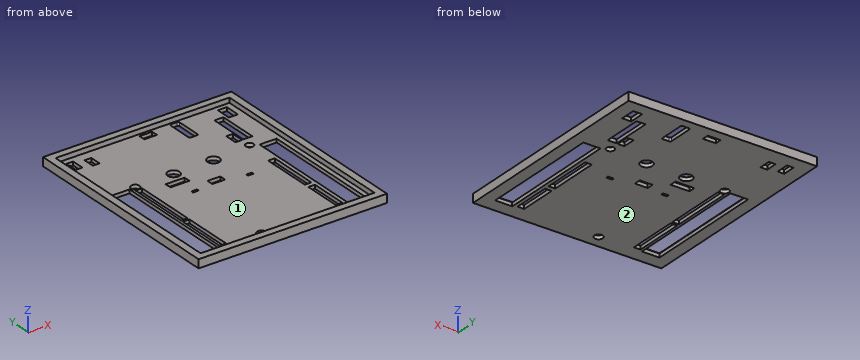
from build123d import *

# Parameters (mm, degrees)
SKETCH1_W           = 78
SKETCH1_H           = 88.5
SKETCH1_W_2         = 72
SKETCH1_H_2         = 82.5
BOSS_EXTRUDE1_DEPTH = 2
SKETCH2_W           = 78
SKETCH2_H           = 88.5
BOSS_EXTRUDE2_DEPTH = 1.5
SKETCH7_W           = 7.279998142
SKETCH7_H           = 50.36
SKETCH7_W_2         = 7.079999996
SKETCH7_H_2         = 50.160000192
CUT_EXTRUDE1_DEPTH  = 15
SKETCH8_R           = 1.738
SKETCH8_R_2         = 1.6
CUT_EXTRUDE2_DEPTH  = 10
SKETCH9_R           = 2.464925529
CUT_EXTRUDE3_DEPTH  = 10
SKETCH11_W          = 5.279999902
SKETCH11_H          = 2.74
SKETCH11_W_2        = 2.74
SKETCH11_H_2        = 5.28
SKETCH11_W_3        = 7.819999902
SKETCH11_W_4        = 5.280000098
SKETCH11_H_3        = 2.739999805
CUT_EXTRUDE4_DEPTH  = 10
SKETCH10_W          = 2.740000978
SKETCH10_H          = 25.907999907
SKETCH10_W_2        = 2.739999218
SKETCH10_H_2        = 20.828000093
SKETCH10_W_3        = 2.73999941
SKETCH10_H_3        = 15.594000099
SKETCH10_W_4        = 3.739999409
SKETCH10_H_4        = 16.440000004
SKETCH10_W_5        = 2.739999409
SKETCH10_H_5        = 15.440000004
SKETCH10_W_6        = 3.739999801
SKETCH10_H_6        = 6.280000102
SKETCH10_W_7        = 2.739999801
SKETCH10_H_7        = 5.280000102
CUT_EXTRUDE5_DEPTH  = 10
CUT_EXTRUDE6_DEPTH  = 10


with BuildPart() as part:
    # Sketch1 → Boss-Extrude1 (new body)
    with BuildSketch(Plane.XY):
        with Locations((19.784172662, -18.690647482)):
            Rectangle(SKETCH1_W, SKETCH1_H)
        with Locations((19.784172662, -18.690647482)):
            Rectangle(SKETCH1_W_2, SKETCH1_H_2, mode=Mode.SUBTRACT)
    extrude(amount=BOSS_EXTRUDE1_DEPTH)

    # Sketch2 → Boss-Extrude2 (add)
    with BuildSketch(Plane(origin=(0, 0, 0), x_dir=(-1, 0, 0), z_dir=(0, 0, -1))):
        with Locations((-19.784172662, -18.690647482)):
            Rectangle(SKETCH2_W, SKETCH2_H)
    extrude(amount=BOSS_EXTRUDE2_DEPTH)

    # Sketch7 → Cut-Extrude1 (cut)
    with BuildSketch(Plane.XY):
        with Locations((-10.583804942, -31.990645157)):
            Rectangle(SKETCH7_W, SKETCH7_H)
        with Locations((50.276195985, -32.090647407)):
            Rectangle(SKETCH7_W_2, SKETCH7_H_2)
    extrude(amount=-CUT_EXTRUDE1_DEPTH, mode=Mode.SUBTRACT)

    # Sketch8 → Cut-Extrude2 (cut)
    with BuildSketch(Plane(origin=(0, 0, -1.5), x_dir=(-1, 0, 0), z_dir=(0, 0, -1))):
        with Locations((-10.782151243, -57.440646574)):
            Circle(SKETCH8_R)
        with Locations((4.457850712, -6.640647161)):
            Circle(SKETCH8_R)
        with Locations((-43.802149239, -5.370645303)):
            Circle(SKETCH8_R_2)
    extrude(amount=-CUT_EXTRUDE2_DEPTH, mode=Mode.SUBTRACT)

    # Sketch9 → Cut-Extrude3 (cut)
    with BuildSketch(Plane(origin=(0, 0, -1.5), x_dir=(-1, 0, 0), z_dir=(0, 0, -1))):
        with Locations((-27.927151828, -6.640645914)):
            Circle(SKETCH9_R)
        with Locations((-11.417149288, -6.64064655)):
            Circle(SKETCH9_R)
    extrude(amount=-CUT_EXTRUDE3_DEPTH, mode=Mode.SUBTRACT)

    # Sketch11 → Cut-Extrude4 (cut)
    with BuildSketch(Plane(origin=(0, 0, -1.5), x_dir=(-1, 0, 0), z_dir=(0, 0, -1))):
        with Locations((-20.306157662, 20.028363095)):
            Rectangle(SKETCH11_W, SKETCH11_H)
        with Locations((-42.531158468, 1.615345297)):
            Rectangle(SKETCH11_W_2, SKETCH11_H_2)
        with Locations((-8.877149508, -12.355646794)):
            Rectangle(SKETCH11_W_3, SKETCH11_H)
        with Locations((-20.308140255, -18.704655608)):
            Rectangle(SKETCH11_W_4, SKETCH11_H_3)
        with Locations((12.078842143, 17.490343195)):
            Rectangle(SKETCH11_W_2, SKETCH11_H_2)
    extrude(amount=-CUT_EXTRUDE4_DEPTH, mode=Mode.SUBTRACT)

    # Sketch10 → Cut-Extrude5 (cut)
    # profile 1 of 10: a face of its own
    with BuildSketch(Plane(origin=(0, 0, -1.5), x_dir=(-1, 0, 0), z_dir=(0, 0, -1))):
        with Locations((4.457850135, -21.62664716)):
            Rectangle(SKETCH10_W, SKETCH10_H)
    # profile 2 of 10: a face of its own
    with BuildSketch(Plane(origin=(0, 0, -1.5), x_dir=(-1, 0, 0), z_dir=(0, 0, -1))):
        with Locations((4.457849197, -46.01064716)):
            Rectangle(SKETCH10_W_2, SKETCH10_H_2)
    # profile 3 of 10: a face of its own
    with BuildSketch(Plane(origin=(0, 0, -1.5), x_dir=(-1, 0, 0), z_dir=(0, 0, -1))):
        with Locations((-43.802150903, -48.473645307)):
            Rectangle(SKETCH10_W_3, SKETCH10_H_3)
    # profile 4 of 10: a face of its own
    with BuildSketch(Plane(origin=(0, 0, -1.5), x_dir=(-1, 0, 0), z_dir=(0, 0, -1))):
        with Locations((-43.802150119, -28.230645304)):
            Rectangle(SKETCH10_W_2, SKETCH10_H_2)
    # profile 5 of 10: a face of its own
    with BuildSketch(Plane(origin=(0, 0, -1.5), x_dir=(-1, 0, 0), z_dir=(0, 0, -1))):
        with Locations((-46.342148749, 7.329354744)):
            Rectangle(SKETCH10_W_4, SKETCH10_H_4)
        with Locations((-46.342148749, 7.329354744)):
            Rectangle(SKETCH10_W_5, SKETCH10_H_5, mode=Mode.SUBTRACT)
    # profile 6 of 10: a face of its own
    with BuildSketch(Plane(origin=(0, 0, -1.5), x_dir=(-1, 0, 0), z_dir=(0, 0, -1))):
        with Locations((-46.342148749, 7.329354744)):
            Rectangle(SKETCH10_W_5, SKETCH10_H_5)
    # profile 7 of 10: a face of its own
    with BuildSketch(Plane(origin=(0, 0, -1.5), x_dir=(-1, 0, 0), z_dir=(0, 0, -1))):
        with Locations((-51.421157761, 17.490345588)):
            Rectangle(SKETCH10_W_6, SKETCH10_H_6)
        with Locations((-51.421157761, 17.490345588)):
            Rectangle(SKETCH10_W_7, SKETCH10_H_7, mode=Mode.SUBTRACT)
    # profile 8 of 10: a face of its own
    with BuildSketch(Plane(origin=(0, 0, -1.5), x_dir=(-1, 0, 0), z_dir=(0, 0, -1))):
        with Locations((-51.421157761, 17.490345588)):
            Rectangle(SKETCH10_W_7, SKETCH10_H_7)
    # profile 9 of 10: a face of its own
    with BuildSketch(Plane(origin=(0, 0, -1.5), x_dir=(-1, 0, 0), z_dir=(0, 0, -1))):
        with BuildLine():
            Line((-31.10214819, 21.899354208), (-33.64214819, 21.899354306))
            ThreePointArc((-33.64214819, 21.899354306), (-34.066412265, 21.723618391), (-34.242148213, 21.299354329))
            Line((-34.242148213, 21.299354329), (-34.242148604, 11.139354329))
            ThreePointArc((-34.242148604, 11.139354329), (-34.066412689, 10.715090253), (-33.642148627, 10.539354306))
            Line((-33.642148627, 10.539354306), (-31.102148627, 10.539354208))
            ThreePointArc((-31.102148627, 10.539354208), (-30.677884552, 10.715090123), (-30.502148604, 11.139354185))
            Line((-30.502148604, 11.139354185), (-30.502148213, 21.299354185))
            ThreePointArc((-30.502148213, 21.299354185), (-30.677884128, 21.72361826), (-31.10214819, 21.899354208))
        make_face()
        with BuildLine():
            ThreePointArc((-33.742148604, 11.139354309), (-33.712859285, 11.06864363), (-33.642148608, 11.039354306))
            Line((-33.642148608, 11.039354306), (-31.102148608, 11.039354208))
            ThreePointArc((-31.102148608, 11.039354208), (-31.031437929, 11.068643527), (-31.002148604, 11.139354204))
            Line((-31.002148604, 11.139354204), (-31.002148213, 21.299354204))
            ThreePointArc((-31.002148213, 21.299354204), (-31.031437532, 21.370064883), (-31.102148209, 21.399354208))
            Line((-31.102148209, 21.399354208), (-33.642148209, 21.399354306))
            ThreePointArc((-33.642148209, 21.399354306), (-33.712858888, 21.370064986), (-33.742148213, 21.299354309))
            Line((-33.742148213, 21.299354309), (-33.742148604, 11.139354309))
        make_face(mode=Mode.SUBTRACT)
    # profile 10 of 10: a face of its own
    with BuildSketch(Plane(origin=(0, 0, -1.5), x_dir=(-1, 0, 0), z_dir=(0, 0, -1))):
        with BuildLine():
            Line((-33.742148213, 21.299354309), (-33.742148604, 11.139354309))
            ThreePointArc((-33.742148604, 11.139354309), (-33.712859285, 11.06864363), (-33.642148608, 11.039354306))
            Line((-33.642148608, 11.039354306), (-31.102148608, 11.039354208))
            ThreePointArc((-31.102148608, 11.039354208), (-31.031437929, 11.068643527), (-31.002148604, 11.139354204))
            Line((-31.002148604, 11.139354204), (-31.002148213, 21.299354204))
            ThreePointArc((-31.002148213, 21.299354204), (-31.031437532, 21.370064883), (-31.102148209, 21.399354208))
            Line((-31.102148209, 21.399354208), (-33.642148209, 21.399354306))
            ThreePointArc((-33.642148209, 21.399354306), (-33.712858888, 21.370064986), (-33.742148213, 21.299354309))
        make_face()
    extrude(amount=-CUT_EXTRUDE5_DEPTH, mode=Mode.SUBTRACT)

    # Sketch12 → Cut-Extrude6 (cut)
    with BuildSketch(Plane(origin=(0, 0, -1.5), x_dir=(-1, 0, 0), z_dir=(0, 0, -1))):
        Polygon((-33.108749893, -22.363499715), (-32.143549893, -22.363499752), (-30.746549856, -22.363499715), (-30.746549856, -21.398299806), (-31.711749856, -21.398299769), (-33.108749893, -21.398299806), align=None)
        Polygon((-11.328249844, -20.128046644), (-11.328249844, -21.093246553), (-10.363049844, -21.09324659), (-8.966049807, -21.093246553), (-8.966049807, -20.128046644), (-9.931249807, -20.128046607), align=None)
        Polygon((4.326251742, 13.867754697), (5.826253641, 13.867754697), (7.129451441, 13.867754697), (7.129451441, 18.570950884), (5.629449542, 18.570950884), (4.326251742, 18.570950884), align=None)
    extrude(amount=-CUT_EXTRUDE6_DEPTH, mode=Mode.SUBTRACT)


solid = part.part
Source: CAD feature listing. Evaluate the final solid. Frame: model axes, mm. Face numbers are marked on the shaded views. Round coordinates to 2 decimals unless told otherwise and drop trailing zeros. Order: outer loops, then holes, each group sorted by start corner. A loop starts at its lowest first (then second) coordinate and runs counter-clockwise, first axis right, second up. Notation, with made-up numbers: (-16, -29.5) - (9, -29.5) arc R12 cw to (9, -13.5) - close; hole circle Ø4 at (18, 74). An arc over 180 degrees is marked (long way). Use a Markdown table: item, result. Add a question column.
1. Section query B-B (y = -51.5). Return the cut outline in (x, z).
2. First-contact query: pin 1 (5 mm diameter, centred on x = -4.5, y = -48, fed in from +Z). Flat tip, straight axial feed; report the tip coordinate or a pass-through.
3. Line query: probe 1 along X at (y, z) = (-42, -0.2); probe 2 along X at (y, z) = (-21, -0.9); probe 3 along X at (y, z) = (-13.5, -1). Output: solid intervals per line, ascending.
4. Section query D-D (y = 9.5). Return the cut outline in (x, z), then the cut area to 3 significant figures.
5. Section query C-C (x = 3.5). Return the cut outline in (y, z), then the cut area to 3 significant figures.
6. Section query A-A (z = 0.65). Return the cut outline in (x, y), then the cut area to 3 significant figures.
7. Mould query, pull axis Y, two halves, no side actions, for the marked faces 1 and 2. Classes: +Y half, -Y half, draft (parallel to the pull), parting line (faces both ways), or undercut.
Derived:
| question | item | result |
|---|---|---|
| 1 | outline | (-19.22, -1.5) - (-14.22, -1.5) - (-14.22, 0) - (-16.22, 0) - (-16.22, 2) - (-19.22, 2) - close; (-6.94, -1.5) - (-5.83, -1.5) - (-5.83, 0) - (-6.94, 0) - close; (-3.09, -1.5) - (42.43, -1.5) - (42.43, 0) - (-3.09, 0) - close; (45.17, -1.5) - (46.74, -1.5) - (46.74, 0) - (45.17, 0) - close; (53.82, -1.5) - (58.78, -1.5) - (58.78, 2) - (55.78, 2) - (55.78, 0) - (53.82, 0) - close |
| 2 | pin 1 | z = 0 |
| 3 | probe 1 | -19.22 to -14.22, -6.94 to -5.83, -3.09 to 42.43, 45.17 to 46.74, 53.82 to 58.78 |
| 3 | probe 2 | -19.22 to -14.22, -6.94 to -5.83, -3.09 to 8.97, 11.33 to 42.43, 45.17 to 46.74, 53.82 to 58.78 |
| 3 | probe 3 | -19.22 to -14.22, -6.94 to -5.83, -3.09 to 4.97, 12.79 to 46.74, 53.82 to 58.78 |
| 4 | outline | (-19.22, -1.5) - (44.47, -1.5) - (44.47, 0) - (-16.22, 0) - (-16.22, 2) - (-19.22, 2) - close; (48.21, -1.5) - (58.78, -1.5) - (58.78, 2) - (55.78, 2) - (55.78, 0) - (48.21, 0) - close |
| 4 | area | 123 mm2 |
| 5 | outline | (-62.94, -1.5) - (25.56, -1.5) - (25.56, 2) - (22.56, 2) - (22.56, 0) - (-59.94, 0) - (-59.94, 2) - (-62.94, 2) - close |
| 5 | area | 145 mm2 |
| 6 | outline | (-19.22, -62.94) - (58.78, -62.94) - (58.78, 25.56) - (-19.22, 25.56) - close; hole (-16.22, -59.94) - (55.78, -59.94) - (55.78, 22.56) - (-16.22, 22.56) - close |
| 6 | area | 963 mm2 |
| 7 | face 1 | undercut |
| 7 | face 2 | draft |
